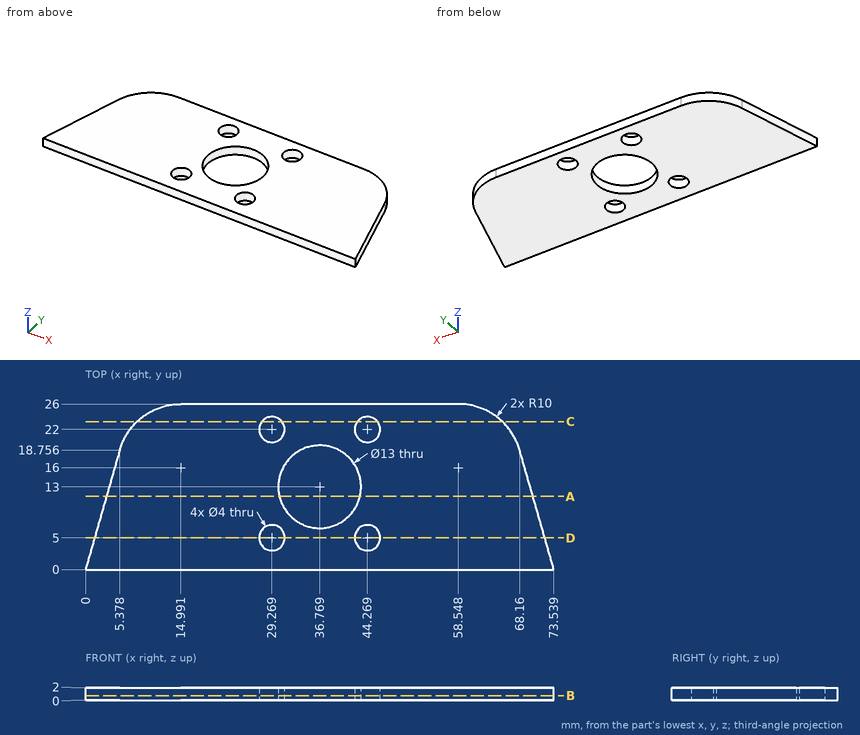
Answer from the drawing. Dimensions are ordinates in mm from the lowest x, y and z of the part. Round coordinates to 2 decimals unless told otherwise and drop trailing zeros. Write each loop counter-clockwise with the first axis right and the second up, starting at its lowest first coordinate (ties: lowest second). Pieces come first, ordered by that corner, then holes.
1. The part is cut by section B-B, the plane z = 0.75. Determine the outline of the cut face in (x, y).
2. The part is cut by section C-C, the plane y = 23.25. Determine the outline of the cut face in (x, z) (1 decimal).
3. The part is cut by section D-D, the plane y = 5. Determine the outline of the cut face in (x, z) (1 decimal), then the cut area to 3 significant figures.
4. The part is cut by section A-A, the plane y = 11.5. Determine the outline of the cut face in (x, z) (1 decimal), then the cut area to 3 significant figures.
5. Given pin 1 Ø1 at (x, y) = (60.5, 5.5) entering from -Z, flat-ended and moving along its own axis, determine where the tip first touches the part or whether it passes through.
6. Straight lines are drawn through the part: L1, parallel to Y at x = 44.5, z = 1.7; L2, parallel to X at y = 5.5, z = 0.5 (1 decimal); L3, parallel to Y at x = 28, z = 1.2 (1 decimal). For each, find the intervals that lie inside material, in ascending order.
Values:
1. outline: (0, 0) - (73.54, 0) - (68.16, 18.76) arc R10 ccw to (58.55, 26) - (14.99, 26) arc R10 ccw to (5.38, 18.76) - close; hole circle Ø4 at (29.27, 5); hole circle Ø4 at (29.27, 22); hole circle Ø13 at (36.77, 13); hole circle Ø4 at (44.27, 5); hole circle Ø4 at (44.27, 22)
2. outline: (8.1, 0) - (27.7, 0) - (27.7, 2) - (8.1, 2) - close; (30.8, 0) - (42.7, 0) - (42.7, 2) - (30.8, 2) - close; (45.8, 0) - (65.4, 0) - (65.4, 2) - (45.8, 2) - close
3. outline: (1.4, 0) - (27.3, 0) - (27.3, 2) - (1.4, 2) - close; (31.3, 0) - (42.3, 0) - (42.3, 2) - (31.3, 2) - close; (46.3, 0) - (72.1, 0) - (72.1, 2) - (46.3, 2) - close
3. area: 125 mm2
4. outline: (3.3, 0) - (30.4, 0) - (30.4, 2) - (3.3, 2) - close; (43.1, 0) - (70.2, 0) - (70.2, 2) - (43.1, 2) - close
4. area: 109 mm2
5. pin 1: stops at z = 0
6. L1: y = 0 to 3.01, 6.99 to 20.01, 23.99 to 26
6. L2: x = 1.6 to 27.3, 31.2 to 42.3, 46.2 to 72
6. L3: y = 0 to 3.5, 6.5 to 20.5, 23.5 to 26
